from build123d import *

# Parameters (mm, degrees)
BASPROSKE_W         = 4
BASPROSKE_H         = 6
TOOTHCUT_DEPTH      = 10.38083152
TEETHCUTS_COUNT     = 10
TEETHCUTS_ANGLE     = 324
BORSKE_R            = 2.5
BORE_DEPTH          = 50.0000508
SKETCH1_R           = 2.5
BOSS_EXTRUDE1_DEPTH = 4
FILLET1_R           = 0.5


with BuildPart() as part:
    # BasProSke → Base-Revolve (revolve)
    with BuildSketch(Plane(origin=(0, 0, 0), x_dir=(1, 0, 0), z_dir=(0, 1, 0)), mode=Mode.PRIVATE) as base_revolve_sk:
        with Locations((2, 3)):
            Rectangle(BASPROSKE_W, BASPROSKE_H)
    revolve(base_revolve_sk.sketch.rotate(Axis((-10, 0, 0), (1, 0, 0)), 180), axis=Axis((-10, 0, 0), (1, 0, 0)))

    # TooCutSke → ToothCut (cut, through all)
    with BuildSketch(Plane(origin=(0, 0, 0), x_dir=(0, 0, -1), z_dir=(1, 0, 0))):
        with BuildLine():
            ThreePointArc((0.59278292, 3.701838653), (0, 3.749), (-0.59278292, 3.701838653))
            ThreePointArc((-0.59278292, 3.701838653), (-0.846593509, 4.924114224), (-1.775771316, 5.757784417))
            ThreePointArc((-1.775771316, 5.757784417), (0, 6.0254), (1.775771316, 5.757784417))
            ThreePointArc((1.775771316, 5.757784417), (0.846593509, 4.924114224), (0.59278292, 3.701838653))
        make_face()
    toothcut = extrude(amount=TOOTHCUT_DEPTH, mode=Mode.SUBTRACT)

    # TeethCuts: ToothCut ×10 about axis
    teethcuts_axis = Axis((-10, 0, 0), (1, 0, 0))
    for i in range(1, TEETHCUTS_COUNT):
        add(toothcut.rotate(teethcuts_axis, i * TEETHCUTS_ANGLE / (TEETHCUTS_COUNT - 1)), mode=Mode.SUBTRACT)

    # BorSke → Bore (cut, symmetric)
    with BuildSketch(Plane(origin=(0, 0, 0), x_dir=(0, 0, -1), z_dir=(1, 0, 0))):
        with Locations(Location((0, 0, 0), (0, 0, 180))):
            Circle(BORSKE_R)
    extrude(amount=BORE_DEPTH, both=True, mode=Mode.SUBTRACT)

    # Sketch1 → Boss-Extrude1 (add)
    with BuildSketch(Plane(origin=(4, 0, 0), x_dir=(0, 0, -1), z_dir=(1, 0, 0))):
        Circle(SKETCH1_R)
        with BuildLine():
            Line((-1.118033989, 1), (1.118033989, 1))
            ThreePointArc((1.118033989, 1), (0, -1.5), (-1.118033989, 1))
        make_face(mode=Mode.SUBTRACT)
    extrude(amount=-BOSS_EXTRUDE1_DEPTH)

    # Fillet1
    fillet1_edges = [part.edges().sort_by_distance(p)[0] for p in [
        (0, 1, 0),
        (4, 1, 0),
        (0, -1.5, 0),
        (4, -1.5, 0),
    ]]
    fillet(fillet1_edges, radius=FILLET1_R)


solid = part.part
Could you check a few things on this model? Use its own coordinates, in mm. Coordinates: 2 decimals unless noted, no trailing zeros. Loops run counter-clockwise (first coordinate to the right, second up) from the corner with the lowest first, then second, coordinate; pieces in that order, holes last.
1. We'd pull the mould along Y, two halves only. Please class faces 1 (the face through (1.972, -2.3, 4.397)), 2 (the face through (1.97, 1.17, 3.56)): released by +Y, released by -Y, zero draft, split by the parting line, or undercut.
2. Imagine slicing it at A-A (z = 0). Please give me the cut outline in (x, y), and give its area (3 significant figures).
3. I need wall thicknesses on L1, parallel to Y at x = 2.5, z = 0; L2, parallel to Z at x = 0.9, y = -4.75; L3, parallel to Z at x = 1.65, y = 0. Which ranges of each line are inside material? Lowest first, please.
4. Imagine slicing it at B-B (z = 3.5). Please give me the cut outline in (x, y).
5. For P1, Ø1, axis at x = 3, y = 2.5, coming from the -Z side; P2, Ø2, axis at y = 4.5, z = 4, coming from the -X side; P3, Ø0.7, axis at x = 2, z = -0.5, coming from the -Y side, each with a flat end and sliding along its axis, tell me the tip position at first contact or that it passes through.
6. Imagine slicing it at C-C (y = 4.5). Please give me the cut outline in (x, z).
7. Imagine slicing it at D-D (z = -4.25). Please give me the cut outline in (x, y), and give its area (3 significant figures).
Computed values:
1. face 1: undercut
1. face 2: undercut
2. outline: (0, -3.75) - (4, -3.75) - (4, -2) arc R0.5 ccw to (3.5, -1.5) - (0.5, -1.5) arc R0.5 ccw to (0, -2) - close; (0, 1.5) arc R0.5 ccw to (0.5, 1) - (3.5, 1) arc R0.5 ccw to (4, 1.5) - (4, 3.75) - (0, 3.75) - close
2. area: 19.8 mm2
3. L1: y = -3.75 to -1.5, 1 to 3.75
3. L2: z = -2.22 to -0.76, 0.76 to 2.22
3. L3: z = -6 to -1.5, 1.5 to 6
4. outline: (0, -3.45) - (4, -3.45) - (4, -1.75) - (0, -1.75) - close; (0, -1.34) - (4, -1.34) - (4, 1.34) - (0, 1.34) - close; (0, 1.75) - (4, 1.75) - (4, 3.45) - (0, 3.45) - close
5. P1: stops at z = -4.82
5. P2: stops at x = 0
5. P3: stops at y = -4.93
6. outline: (0, -2.21) - (4, -2.21) - (4, -0.66) - (0, -0.66) - close; (0, 0.66) - (4, 0.66) - (4, 2.21) - (0, 2.21) - close
7. outline: (0, -3.65) - (4, -3.65) - (4, -2.16) - (0, -2.16) - close; (0, -0.74) - (4, -0.74) - (4, 0.74) - (0, 0.74) - close; (0, 2.16) - (4, 2.16) - (4, 3.65) - (0, 3.65) - close
7. area: 17.9 mm2
